Autodesk Inventor part; units mm, degrees
ref_plane "YZ Plane" through (0, 0, 0) normal (1, 0, 0) x (0, 1, 0)
ref_plane "XZ Plane" through (0, 0, 0) normal (0, 1, 0) x (-1, 0, 0)
ref_plane "XY Plane" through (0, 0, 0) normal (0, 0, 1) x (1, 0, 0)
sketch "Block1" plane through (0, 0, 0) normal (0, 0, 1) x (1, 0, 0)
  circle A0 centre (74.029, 24.2723) radius 1
  line L0 (49.279, 30.4723) -> (71.779, 30.4723)
  line L1 (71.779, 30.4723) -> (71.779, 18.0723)
  line L2 (71.779, 18.0723) -> (49.279, 18.0723)
  line L3 (49.279, 18.0723) -> (49.279, 30.4723)
  line L4 (49.279, 30.4723) -> (44.779, 30.4723)
  line L5 (44.779, 30.4723) -> (44.779, 18.0723)
  line L6 (44.779, 18.0723) -> (49.279, 18.0723)
  line L7 (49.279, 18.0723) -> (49.279, 30.4723)
  line L8 (71.779, 30.4723) -> (76.279, 30.4723)
  line L9 (76.279, 30.4723) -> (76.279, 18.0723)
  line L10 (76.279, 18.0723) -> (71.779, 18.0723)
  line L11 (71.779, 18.0723) -> (71.779, 30.4723)
  line L12 (44.779, 24.2723) -> (76.279, 24.2723) construction
  line L13 (47.029, 30.4723) -> (47.029, 18.0723) construction
  circle A1 centre (47.029, 24.2723) radius 1
  line L14 (74.029, 30.4723) -> (74.029, 18.0723) construction
  point P0 (60.979, 24.0984)
  dimension "d7" = 22.5
  dimension "d8" = 12.4
  dimension "d9" = 4.5
  dimension "d10" = 4.5
  dimension "d11" = 2
  dimension "d12" = 2
sketch "Sketch1" plane through (0, 0, 0) normal (0, 0, 1) x (1, 0, 0)
  line L0 (-92.7646, -8.503) -> (-89.7646, -8.503)
  line L1 (-89.7646, -8.503) -> (-89.7646, -11.753)
  line L2 (-89.7646, -11.753) -> (-92.7646, -11.753)
  line L3 (-92.7646, -11.753) -> (-92.7646, -8.503)
  line L4 (-92.7646, -21.6527) -> (-89.7646, -21.6527)
  line L5 (-89.7646, -21.6527) -> (-89.7646, -21.7527)
  line L6 (-89.7646, -21.7527) -> (-92.7646, -21.7527)
  line L7 (-92.7646, -21.7527) -> (-92.7646, -21.6527)
  line L8 (-27.4321, 29.4262) -> (-8.6821, 29.4262)
  line L9 (-8.6821, 29.4262) -> (-8.6821, 11.4262)
  line L10 (-8.6821, 11.4262) -> (-27.4321, 11.4262)
  line L11 (-27.4321, 11.4262) -> (-27.4321, 29.4262)
  line L12 (-27.4321, 20.4262) -> (-8.6821, 20.4262) construction
  line L13 (-30.6821, 27.4262) -> (-27.4321, 27.4262)
  line L14 (-27.4321, 27.4262) -> (-27.4321, 13.4262)
  line L15 (-27.4321, 13.4262) -> (-30.6821, 13.4262)
  line L16 (-30.6821, 13.4262) -> (-30.6821, 27.4262)
  line L17 (-30.6821, 20.4262) -> (-27.4321, 20.4262) construction
  line L18 (-18.0571, 29.4262) -> (-18.0571, 11.4262) construction
  line L19 (-5.4321, 27.4262) -> (-8.6821, 27.4262)
  line L20 (-8.6821, 27.4262) -> (-8.6821, 13.4262)
  line L21 (-8.6821, 13.4262) -> (-5.4321, 13.4262)
  line L22 (-5.4321, 13.4262) -> (-5.4321, 27.4262)
  line L23 (-5.4321, 20.4262) -> (-8.6821, 20.4262) construction
  point P0 (0, 0)
  dimension "d0" = 3
  dimension "mat" = 3.25
  dimension "d2" = 3
  dimension "d3" = 0.1
  dimension "d36" = 18.75
  dimension "d37" = 18
  dimension "d38" = 3.25
  dimension "d39" = 14
extrude "Extrusion4" add sketch "Sketch1" along normal blind 3.25 contours L8 L9 L10 L11 | L11 L15 L16 L13 | L19 L22 L21 L9
equation "\"d38\" = mat"
equation "\"d40\" = mat"
properties part number "arm-servo"
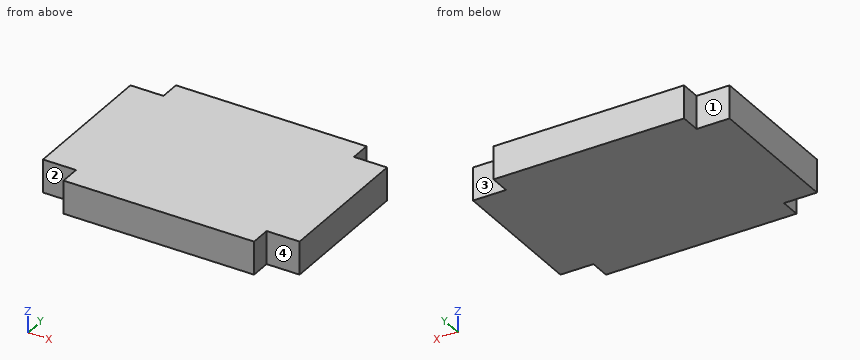
Part model, mm, in its own coordinate system. Face numbers are marked on the shaded views. A direction names the side the tool comes from. Give positions to 0.01 mm unless a question says otherwise; leave off trailing zeros. Order: outer loops, then holes, each group sorted by start corner. A loop starts at its lowest first (then second) coordinate and runs counter-clockwise, first axis right, second up. Notation, with made-up numbers: M 46,28.5 L 90,28.5 A21 ccw 90,49.5 Z; hole C -8,10 d2. An arc over 180 degrees is marked long. Use a Markdown table: item, result. Add a question column.
(1) 3-axis set-ups, long thin cutter, end or side, ignore diameter. For the marked faces 1, 2, 3 and 4: which of +Z, -Z, +X, -X, +Y, -Y reach the whole face in a straight line?
(2) Saw through at B-B, the plane x = -7. Give the cut face in (y, z).
(3) Probe line 1 along Y through (x, z) = (-6.5, 2.95); line 2 along X through (y, z) = (13.25, 1.85). List the from-to ranges inside material, lowest first. Write a range as [from, to].
(4) Drop flat-ended pins along their axis: P1, Ø1, axis at y = 28, z = 1.5, coming from the -X side; P2, Ø1.6, axis at x = -29.5, z = 1.5, coming from the +Y side; P3, Ø1, axis at y = 13, z = 2, coming from the -X side; P4, Ø1.6, axis at y = 29, z = 2, coming from the +X side. Give the stop position or say it passes through.
(5) Saw through at C-C, the plane y = 28.25. Give the cut face in (x, z).
(6) Saw through at A-A, the plane z = 2.15. Give the cut face in (x, y), and give its area (4 significant figures).
Answer key:
| question | item | result |
|---|---|---|
| 1 | face 1 | +Z, -Z, -X, +Y |
| 1 | face 2 | +Z, -Z, -X, -Y |
| 1 | face 3 | +Z, -Z, +X, +Y |
| 1 | face 4 | +Z, -Z, +X, -Y |
| 2 | outline | M 13.43,0 L 27.43,0 L 27.43,3.25 L 13.43,3.25 Z |
| 3 | line 1 | [13.43, 27.43] |
| 3 | line 2 | [-27.43, -8.68] |
| 4 | P1 | x = -27.43 |
| 4 | P2 | y = 27.43 |
| 4 | P3 | x = -30.68 |
| 4 | P4 | x = -8.68 |
| 5 | outline | M -27.43,0 L -8.68,0 L -8.68,3.25 L -27.43,3.25 Z |
| 6 | outline | M -30.68,13.43 L -27.43,13.43 L -27.43,11.43 L -8.68,11.43 L -8.68,13.43 L -5.43,13.43 L -5.43,27.43 L -8.68,27.43 L -8.68,29.43 L -27.43,29.43 L -27.43,27.43 L -30.68,27.43 Z |
| 6 | area | 428.5 mm^2 |
